Could you check a few things on this model? Use its own coordinates, in mm. Round coordinates to 2 decimals unless told otherwise and drop trailing zeros. Write each loop counter-clockwise with the first axis right and the second up, starting at its lowest first coordinate (ties: lowest second). Pieces come first, ordered by that corner, then holes. Notation, with made-up numbers: (-38.75, 7) -> (11.25, 7) arc R6 ccw to (11.25, 13) -> close; hole circle Ø8 at (-35, 17.25). An arc over 180 degrees is marked (long way). One line per question, with ' | ' between items. Start each with the question number.
1. Imagine slicing it at B-B, the plane y = -21.5. List the corners of the cut face in (x, z) for me, and give its area (3 significant figures).
2. If I drill on line 1 along X through (y, z) = (-21.25, 3.75); line 2 along X through (y, z) = (-17.75, 6); line 3 along Y through (x, z) = (-182.5, 4.75), over which ranges is the centre line in solid material (lowest first)? Write a range as [from, to].
3. Imagine slicing it at C-C, the plane x = -184. List the corners of the cut face in (y, z) for me, and give its area (3 significant figures).
4. For pin 1 Ø1.5 at (x, z) = (-197.5, 7) entering from +Y, with a flat end and sliding along its axis, tell me the tip position at first contact or that it passes through.
5. Imagine slicing it at A-A, the plane z = 0.75. List the corners of the cut face in (x, y) for me, and give its area (3 significant figures).
from build123d import *

# Parameters (mm, degrees)
EXTRUDE_1_DEPTH     = 8
SKETCH_2_W          = 25.296907813
SKETCH_2_H          = 21.985442263
SKETCH_2_W_2        = 19.585718922
SKETCH_2_H_2        = 21.456908972
CUT_EXTRUDE_1_DEPTH = 215.146433821


with BuildPart() as part:
    # Эскиз1 → Вытянуть1 (new body)
    with BuildSketch(Plane.XY):
        Polygon((-210.000000639, 0), (-210.000000639, -41.166671594), (-156.500000575, 0), align=None)
    extrude(amount=EXTRUDE_1_DEPTH)

    # Эскиз2 → Вырез-Вытянуть1 (cut, through all)
    with BuildSketch(Plane.XY.offset(8)):
        with Locations((-197.351546733, -34.775510048)):
            Rectangle(SKETCH_2_W, SKETCH_2_H)
        with Locations((-166.292859318, -6.126894901)):
            Rectangle(SKETCH_2_W_2, SKETCH_2_H_2)
    extrude(amount=-CUT_EXTRUDE_1_DEPTH, mode=Mode.SUBTRACT)


solid = part.part
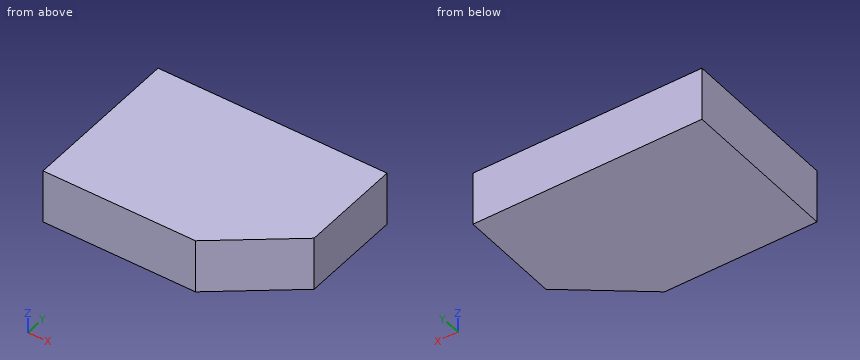
Geometry results:
1) outline: (-210, 0) -> (-184.44, 0) -> (-184.44, 8) -> (-210, 8) -> close | area: 204 mm2
2) line 1: x = [-210, -184.12] | line 2: x = [-210, -179.57] | line 3: y = [-20.01, 0]
3) outline: (-21.16, 0) -> (0, 0) -> (0, 8) -> (-21.16, 8) -> close | area: 169 mm2
4) pin 1: stops at y = 0
5) outline: (-210, -23.78) -> (-187.41, -23.78) -> (-176.09, -15.07) -> (-176.09, 0) -> (-210, 0) -> close | area: 757 mm2
